Source: three-view drawing plus pictorial views. Frame: mm from the lowest corner of the part. A direction names the side the tool comes from. Give positions to 0.01 mm unless a question says otherwise; leave off trailing zeros. Write each loop counter-clockwise with the first axis right and the second up, starting at its lowest first coordinate (ties: lowest second). Pieces come first, ordered by that corner, then holes.
Q1. Line query: L1, parallel to X at y = 25.75, z = 5.25; L2, parallel to X at y = 4.75, z = 4 (1 decimal); L3, parallel to X at y = 8.5, z = 9.25. Output: solid intervals per line, ascending.
Q2. Draft query along X for the marked faces 4, 5 and 6. Return one class per face: pulls with the +X half, pulls with the -X half, needs draft (parallel to the pull), parting line crosses it, or undercut.
Q3. Cut plane B-B on y = 9. Return the cut outline in (x, z), plus the area to 3 significant figures.
Q4. Cut plane A-A on y = 27.75. Return the cut outline in (x, z), plus the area to 3 significant figures.
Q5. Cut plane C-C on z = 3. Return the cut outline in (x, y).
Q6. Pin query (flat end, axial travel): pin 1 (3 mm diameter, centred on y = 6.5, z = 3.5, fed in from -X); pin 2 (3 mm diameter, centred on x = 33, z = 6.5, fed in from +Y). Return the tip coordinate at first contact, or that it passes through.
Q7. Cut plane D-D on x = 23.5. Return the cut outline in (y, z).
Q8. Reachability of the marked faces 1, 2 and 3 from +Z, -Z, +X, -X, +Y, -Y: full face, straight path, thin tool, end or side. Return the list, or none.
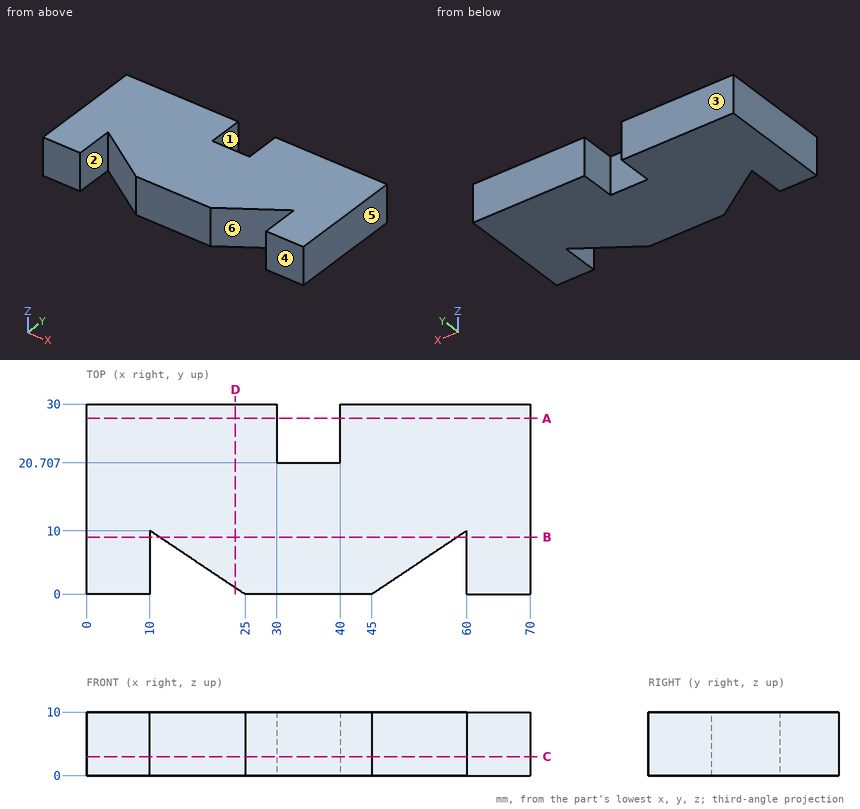
Data:
1. L1: x = 0 to 30, 40 to 70
1. L2: x = 0 to 10, 17.9 to 52.1, 60 to 70
1. L3: x = 0 to 10, 12.25 to 57.75, 60 to 70
2. face 4: needs draft
2. face 5: pulls with the +X half
2. face 6: undercut
3. outline: (0, 0) - (10, 0) - (10, 10) - (0, 10) - close; (11.5, 0) - (58.5, 0) - (58.5, 10) - (11.5, 10) - close; (60, 0) - (70, 0) - (70, 10) - (60, 10) - close
3. area: 670 mm2
4. outline: (0, 0) - (30, 0) - (30, 10) - (0, 10) - close; (40, 0) - (70, 0) - (70, 10) - (40, 10) - close
4. area: 600 mm2
5. outline: (0, 0) - (10, 0) - (10, 10) - (25, 0) - (45, 0) - (60, 10) - (60, 0) - (70, 0) - (70, 30) - (40, 30) - (40, 20.71) - (30, 20.71) - (30, 30) - (0, 30) - close
6. pin 1: stops at x = 0
6. pin 2: stops at y = 20.71
7. outline: (1, 0) - (30, 0) - (30, 10) - (1, 10) - close
8. face 1: +Z, -Z, +Y
8. face 2: +Z, -Z, -Y
8. face 3: +Z, -Z, +X, -X, +Y
